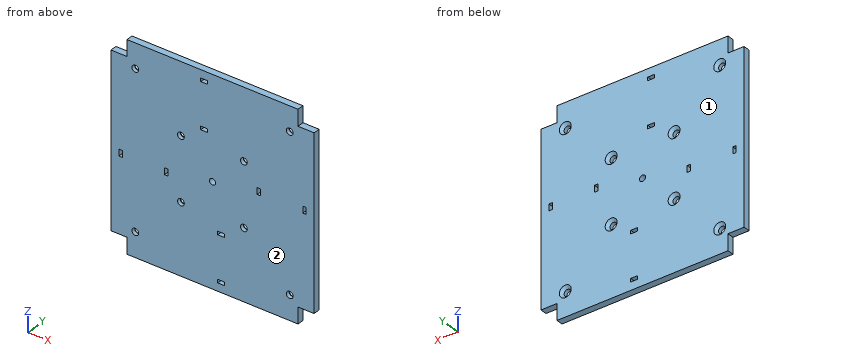
from build123d import *

# Parameters (mm, degrees)
SKETCH1_W                                     = 98
SKETCH1_H                                     = 98
BOSS_EXTRUDE1_DEPTH                           = 3.175
SKETCH2_W                                     = 7.5
SKETCH2_H                                     = 7.5
CUT_EXTRUDE1_DEPTH                            = 70.369161917
F_4_CLEARANCE_HOLE1_D                         = 2.9464
CSK_FOR_4_FLAT_HEAD_MACHINE_SCREW1_AT_2_COUNT = 2
CSK_FOR_4_FLAT_HEAD_MACHINE_SCREW1_AT_2_PITCH = 74.5
CSK_FOR_4_FLAT_HEAD_MACHINE_SCREW1_AT_3_COUNT = 2
CSK_FOR_4_FLAT_HEAD_MACHINE_SCREW1_AT_3_PITCH = 105.358910397
CSK_FOR_4_FLAT_HEAD_MACHINE_SCREW1_AT_4_COUNT = 2
CSK_FOR_4_FLAT_HEAD_MACHINE_SCREW1_AT_4_PITCH = 74.5
CSK_FOR_4_FLAT_HEAD_MACHINE_SCREW2_AT_2_COUNT = 2
CSK_FOR_4_FLAT_HEAD_MACHINE_SCREW2_AT_2_PITCH = 30.3784
CSK_FOR_4_FLAT_HEAD_MACHINE_SCREW2_AT_3_COUNT = 2
CSK_FOR_4_FLAT_HEAD_MACHINE_SCREW2_AT_3_PITCH = 42.961545283
CSK_FOR_4_FLAT_HEAD_MACHINE_SCREW2_AT_4_COUNT = 2
CSK_FOR_4_FLAT_HEAD_MACHINE_SCREW2_AT_4_PITCH = 30.3784
CUT_EXTRUDE2_DEPTH                            = 70.369161917
SKETCH16_W                                    = 1.651
SKETCH16_H                                    = 3.175
CUT_EXTRUDE3_DEPTH                            = 70.369161917
CIRPATTERN1_COUNT                             = 4


with BuildPart() as part:
    # Sketch1 → Boss-Extrude1 (new body)
    with BuildSketch(Plane(origin=(0, 0, 0), x_dir=(1, 0, 0), z_dir=(0, 1, 0))):
        Rectangle(SKETCH1_W, SKETCH1_H)
    extrude(amount=BOSS_EXTRUDE1_DEPTH)

    # Sketch2 → Cut-Extrude1 (cut, through all)
    with BuildSketch(Plane(origin=(0, 3.175, 0), x_dir=(1, 0, 0), z_dir=(0, 1, 0))):
        with Locations((45.25, 45.25)):
            Rectangle(SKETCH2_W, SKETCH2_H)
        with Locations((-45.25, 45.25)):
            Rectangle(SKETCH2_W, SKETCH2_H)
        with Locations((45.25, -45.25)):
            Rectangle(SKETCH2_W, SKETCH2_H)
        with Locations((-45.25, -45.25)):
            Rectangle(SKETCH2_W, SKETCH2_H)
    extrude(amount=-CUT_EXTRUDE1_DEPTH, mode=Mode.SUBTRACT)

    # #4 Clearance Hole1 (through all)
    with Locations(Plane(origin=(0, 3.175, 0), x_dir=(1, 0, 0), z_dir=(0, 1, 0))):
        with Locations((0, 0)):
            Hole(F_4_CLEARANCE_HOLE1_D / 2)

    # Sketch9 → CSK for #4 Flat Head Machine Screw1 (revolve, cut)
    with BuildSketch(Plane(origin=(37.25, 3.175, 37.25), x_dir=(0, 0, 1), z_dir=(1, 0, 0))):
        Polygon((0, 0), (0, 3.175), (1.63195, 3.175), (1.63195, 1.409834001), (2.8575, 0), align=None)
    csk_for_4_flat_head_machine_screw1 = revolve(axis=Axis((37.25, 9.525, 37.25), (0, -1, 0)), mode=Mode.SUBTRACT)

    # CSK for #4 Flat Head Machine Screw1 at 2: CSK for #4 Flat Head Machine Screw1 ×2
    with Locations(*[(-i * CSK_FOR_4_FLAT_HEAD_MACHINE_SCREW1_AT_2_PITCH, 0, 0) for i in range(1, CSK_FOR_4_FLAT_HEAD_MACHINE_SCREW1_AT_2_COUNT)]):
        add(csk_for_4_flat_head_machine_screw1, mode=Mode.SUBTRACT)

    # CSK for #4 Flat Head Machine Screw1 at 3: CSK for #4 Flat Head Machine Screw1 ×2
    with Locations(*[Vector(-0.7071067811865502, 0, -0.7071067811865448) * (i * CSK_FOR_4_FLAT_HEAD_MACHINE_SCREW1_AT_3_PITCH) for i in range(1, CSK_FOR_4_FLAT_HEAD_MACHINE_SCREW1_AT_3_COUNT)]):
        add(csk_for_4_flat_head_machine_screw1, mode=Mode.SUBTRACT)

    # CSK for #4 Flat Head Machine Screw1 at 4: CSK for #4 Flat Head Machine Screw1 ×2
    with Locations(*[(0, 0, -i * CSK_FOR_4_FLAT_HEAD_MACHINE_SCREW1_AT_4_PITCH) for i in range(1, CSK_FOR_4_FLAT_HEAD_MACHINE_SCREW1_AT_4_COUNT)]):
        add(csk_for_4_flat_head_machine_screw1, mode=Mode.SUBTRACT)

    # Sketch13 → CSK for #4 Flat Head Machine Screw2 (revolve, cut)
    with BuildSketch(Plane(origin=(15.1384, 3.175, -15.24), x_dir=(0, 0, 1), z_dir=(1, 0, 0))):
        Polygon((0, 0), (0, 3.175), (1.63195, 3.175), (1.63195, 1.409834001), (2.8575, 0), align=None)
    csk_for_4_flat_head_machine_screw2 = revolve(axis=Axis((15.1384, 9.525, -15.24), (0, -1, 0)), mode=Mode.SUBTRACT)

    # CSK for #4 Flat Head Machine Screw2 at 2: CSK for #4 Flat Head Machine Screw2 ×2
    with Locations(*[(-i * CSK_FOR_4_FLAT_HEAD_MACHINE_SCREW2_AT_2_PITCH, 0, 0) for i in range(1, CSK_FOR_4_FLAT_HEAD_MACHINE_SCREW2_AT_2_COUNT)]):
        add(csk_for_4_flat_head_machine_screw2, mode=Mode.SUBTRACT)

    # CSK for #4 Flat Head Machine Screw2 at 3: CSK for #4 Flat Head Machine Screw2 ×2
    with Locations(*[Vector(-0.7071067811865475, 0, 0.7071067811865477) * (i * CSK_FOR_4_FLAT_HEAD_MACHINE_SCREW2_AT_3_PITCH) for i in range(1, CSK_FOR_4_FLAT_HEAD_MACHINE_SCREW2_AT_3_COUNT)]):
        add(csk_for_4_flat_head_machine_screw2, mode=Mode.SUBTRACT)

    # CSK for #4 Flat Head Machine Screw2 at 4: CSK for #4 Flat Head Machine Screw2 ×2
    with Locations(*[(0, 0, i * CSK_FOR_4_FLAT_HEAD_MACHINE_SCREW2_AT_4_PITCH) for i in range(1, CSK_FOR_4_FLAT_HEAD_MACHINE_SCREW2_AT_4_COUNT)]):
        add(csk_for_4_flat_head_machine_screw2, mode=Mode.SUBTRACT)

    # Sketch15 → Cut-Extrude2 (cut, through all)
    with BuildSketch(Plane(origin=(0, 3.175, 0), x_dir=(1, 0, 0), z_dir=(0, 1, 0))):
        Polygon((-48.746, -41.246), (-41.246, -41.246), (-41.246, -48.746), (-41.246, -49), (-41.5, -49), (-41.5, -41.5), (-49, -41.5), (-49, -41.246), align=None)
        Polygon((49, 41.246), (49, 41.5), (41.5, 41.5), (41.5, 49), (41.246, 49), (41.246, 48.746), (41.246, 41.246), (48.746, 41.246), align=None)
        Polygon((41.246, -48.746), (41.246, -41.246), (48.746, -41.246), (49, -41.246), (49, -41.5), (41.5, -41.5), (41.5, -49), (41.246, -49), align=None)
        Polygon((-41.246, 48.746), (-41.246, 41.246), (-48.746, 41.246), (-49, 41.246), (-49, 41.5), (-41.5, 41.5), (-41.5, 49), (-41.246, 49), align=None)
    extrude(amount=-CUT_EXTRUDE2_DEPTH, mode=Mode.SUBTRACT)

    # Sketch16 → Cut-Extrude3 (cut, through all)
    with BuildSketch(Plane.XZ):
        with Locations((-44.3645, -4.0985)):
            Rectangle(SKETCH16_W, SKETCH16_H)
        with Locations((-22.3935, -4.0985)):
            Rectangle(SKETCH16_W, SKETCH16_H)
    cut_extrude3 = extrude(amount=-CUT_EXTRUDE3_DEPTH, mode=Mode.SUBTRACT)

    # CirPattern1: Cut-Extrude3 ×4 about axis
    cirpattern1_axis = Axis((0, 0, 0), (0, 1, 0))
    for i in range(1, CIRPATTERN1_COUNT):
        add(cut_extrude3.rotate(cirpattern1_axis, i * 360 / CIRPATTERN1_COUNT), mode=Mode.SUBTRACT)


solid = part.part
Here's how the part is built. I have some questions about the finished solid (model axes, mm). Face numbers are marked on the shaded views. Coordinates: 2 decimals unless noted, no trailing zeros. Loops run counter-clockwise (first coordinate to the right, second up) from the corner with the lowest first, then second, coordinate; pieces in that order, holes last. Notation, with made-up numbers: (-1.75, 47) -> (27.25, 47) arc R17 cw to (27.25, 67) -> close; hole circle Ø2 at (71, 48.25). An arc over 180 degrees is marked (long way). Use one line per item in the form item = value. Start each with the question number.
(1) If we section it at A-A (z = 0): Please give me the cut outline in (x, y) (3 decimals).
(2) If we section it at D-D (z = -15.24): Please give me the cut outline in (x, y) (1 decimal).
(3) We'd pull the mould along Y, two halves only. Please class the marked faces 1 and 2: pulls with the +Y half, pulls with the -Y half, needs draft (parallel to the pull), parting line crosses it, or undercut.
(4) Please list where these lines run through material, in increasing order: line 1 along Z through (x, y) = (37.25, 1.4); line 2 along X through (y, z) = (0.5, -3); line 3 along Z through (x, y) = (-38.5, 1.65).
(5) If we section it at C-C (x = 0): Please give me the cut outline in (y, z) (3 decimals).
(6) Will these pins go through, and if not, where does the flat tip stop? pin 1 (0.8 mm diameter, centred on x = -44.5, y = 2, fed in from -Z); pin 2 (5 mm diameter, centred on x = 15.14, z = -15.24, fed in from +Y); pin 3 (1.8 mm diameter, centred on y = 1, z = 44, fed in from +X).
(7) If we section it at B-B (x = -37.25): Please give me the cut outline in (y, z) (1 decimal).
Verdict:
q1.outline = (-49, 0) -> (-1.473, 0) -> (-1.473, 3.175) -> (-49, 3.175) -> close; (1.473, 0) -> (49, 0) -> (49, 3.175) -> (1.473, 3.175) -> close
q2.outline = (-49, 0) -> (-16.9, 0) -> (-16.9, 1.8) -> (-18.1, 3.2) -> (-49, 3.2) -> close; (-13.6, 0) -> (13.5, 0) -> (13.5, 1.8) -> (12.3, 3.2) -> (-12.4, 3.2) -> (-13.6, 1.8) -> close; (16.8, 0) -> (49, 0) -> (49, 3.2) -> (18, 3.2) -> (16.8, 1.8) -> close
q3.face_1 = pulls with the +Y half
q3.face_2 = pulls with the -Y half
q4.line_1 = -49 to -38.88, -35.62 to 35.62, 38.88 to 49
q4.line_2 = -49 to -45.19, -43.54 to -23.22, -21.57 to 49
q4.line_3 = -49 to -38.3, -36.2 to 36.2, 38.3 to 49
q5.outline = (0, -49) -> (3.175, -49) -> (3.175, -1.473) -> (0, -1.473) -> close; (0, 1.473) -> (3.175, 1.473) -> (3.175, 49) -> (0, 49) -> close
q6.pin_1 = -41.25
q6.pin_2 = 2.77
q6.pin_3 = 41.25
q7.outline = (0, -49) -> (3.2, -49) -> (3.2, -40.1) -> (1.8, -38.9) -> (0, -38.9) -> close; (0, -35.6) -> (1.8, -35.6) -> (3.2, -34.4) -> (3.2, 34.4) -> (1.8, 35.6) -> (0, 35.6) -> close; (0, 38.9) -> (1.8, 38.9) -> (3.2, 40.1) -> (3.2, 49) -> (0, 49) -> close
